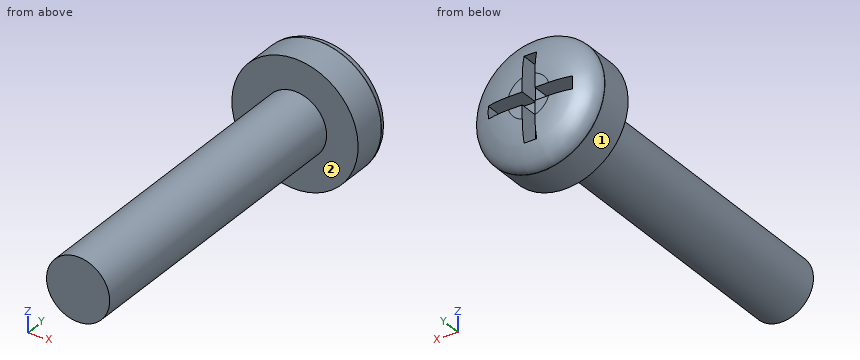
from build123d import *

# Parameters (mm, degrees)
SKICA1_R                 = 1.5
P_IDAT_VYSUNUT_M1_DEPTH  = 15
SKICA2_R                 = 3
P_IDAT_VYSUNUT_M2_DEPTH  = 1.6
SKICA3_R                 = 2.999911278
P_IDAT_VYSUNUT_M3_DEPTH  = 0.92
ZAOBLIT1_SIZE            = 0.9
ZAOBLIT1_SIZE_2          = 2
SKICA4_W                 = 0.6
SKICA4_H                 = 4
SKICA4_W_2               = 4
SKICA4_H_2               = 0.6
ODEBRAT_VYSUNUT_M1_DEPTH = 0.92


with BuildPart() as part:
    # Skica1 → Přidat vysunutím1 (new body)
    with BuildSketch(Plane(origin=(0, 0, 0), x_dir=(1, 0, 0), z_dir=(0, 1, 0))):
        with Locations(Location((0, 0, 0), (0, 0, 270))):
            Circle(SKICA1_R)
    extrude(amount=P_IDAT_VYSUNUT_M1_DEPTH)

    # Skica2 → Přidat vysunutím2 (add)
    with BuildSketch(Plane(origin=(0, 15, 0), x_dir=(1, 0, 0), z_dir=(0, 1, 0))):
        with Locations(Location((0, 0, 0), (0, 0, 270))):
            Circle(SKICA2_R)
    extrude(amount=P_IDAT_VYSUNUT_M2_DEPTH)

    # Skica3 → Přidat vysunutím3 (add)
    with BuildSketch(Plane(origin=(0, 16.6, 0), x_dir=(1, 0, 0), z_dir=(0, 1, 0))):
        with Locations(Location((0, 0, 0), (0, 0, 270))):
            Circle(SKICA3_R)
    extrude(amount=P_IDAT_VYSUNUT_M3_DEPTH)

    # Zaoblit1
    # an asymmetric fillet: 2, 0.9 mm, written as the material it takes off along each edge
    with BuildSketch(Plane(origin=(0, 17.52, 0), x_dir=(0, 0, 1), z_dir=(-1, 0, 0))) as zaoblit1_piece_1:
        with BuildLine():
            Bezier((2.999911278, -ZAOBLIT1_SIZE), (2.999911278, 0), (2.999911278 - ZAOBLIT1_SIZE_2, 0), weights=[1, 0.707106781, 1])
            Line((2.999911278 - ZAOBLIT1_SIZE_2, 0), (2.999911278, 0))
            Line((2.999911278, 0), (2.999911278, -ZAOBLIT1_SIZE))
        make_face()
    revolve(axis=Axis((0, 17.52, 0), (0, 1, 0)), mode=Mode.SUBTRACT)

    # Skica4 → Odebrat vysunutím1 (cut)
    with BuildSketch(Plane(origin=(0, 17.52, 0), x_dir=(1, 0, 0), z_dir=(0, 1, 0))):
        Rectangle(SKICA4_W, SKICA4_H)
        Rectangle(SKICA4_W_2, SKICA4_H_2)
    extrude(amount=-ODEBRAT_VYSUNUT_M1_DEPTH, mode=Mode.SUBTRACT)


solid = part.part
Input: part model. Units: mm. Frame: model coordinates. Face numbers are marked on the shaded views. A direction names the side the tool comes from. Round coordinates to 2 decimals unless told otherwise and drop trailing zeros. Write each loop counter-clockwise with the first axis right and the second up, starting at its lowest first coordinate (ties: lowest second). Pieces come first, ordered by that corner, then holes.
1) Contact query for flat-ended pins moving along their axis: P1, Ø0.7, axis at y = 17, z = 0, coming from the -X side; P2, Ø3, axis at x = -2.5, z = 1.5, coming from the +Y side; P3, Ø0.5, axis at x = 1, y = 17, coming from the +Z side; P4, Ø1, axis at y = 17, z = -1.5, coming from the -X side. Output: stop coordinate, or through.
2) Cut plane B-B (y = 7.5). Return the cut outline in (x, z), then the cut area to 3 significant figures.
3) Ray query, L1, parallel to Y at x = -0.45, z = 0; L2, parallel to Z at x = 0.3, y = 16.5; L3, parallel to Z at x = -0.55, y = 4.5. Return the intervals inside material, ascending.
4) Cut plane A-A (y = 16.25). Return the cut outline in (x, z).
5) Reachability of the marked faces 1 and 2 from +Z, -Z, +X, -X, +Y, -Y: full face, straight path, thin tool, end or side. Return the list, or none.
Geometry says:
1. P1: stops at x = -3
1. P2: stops at y = 17.5
1. P3: stops at z = 2.84
1. P4: stops at x = -2.78
2. outline: circle Ø3 at (0, 0)
2. area: 7.07 mm2
3. L1: y = 0 to 16.6
3. L2: z = -2.98 to 2.98
3. L3: z = -1.4 to 1.4
4. outline: circle Ø6 at (0, 0)
5. face 1: +Y, -Y
5. face 2: -Y
